Source: three-view drawing plus pictorial views. Frame: mm from the lowest corner of the part. A direction names the side the tool comes from. Coordinates: 2 decimals unless noted, no trailing zeros. Write each loop counter-clockwise with the first axis right and the second up, starting at its lowest first coordinate (ties: lowest second). Pieces come first, ordered by that corner, then holes. Notation, with made-up numbers: (-36.5, 71) - (5.5, 71) arc R11 cw to (5.5, 75) - close; hole circle Ø3 at (17.25, 50). An arc over 180 degrees is marked (long way). One line per item, written item: value.
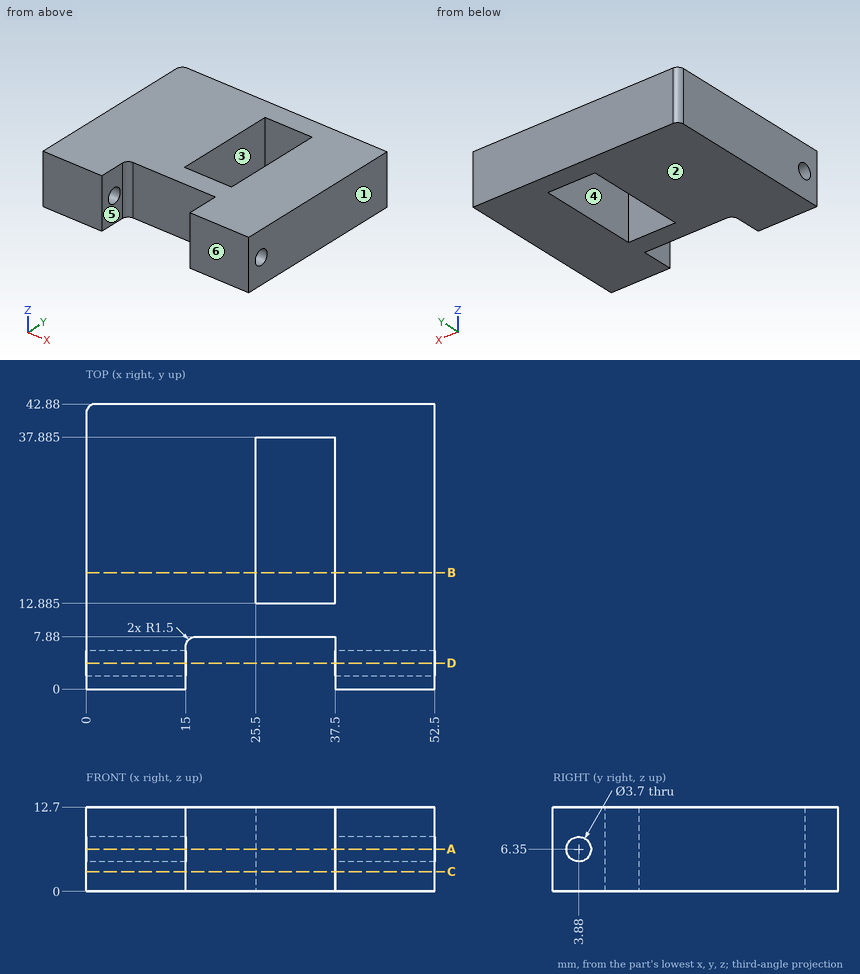
1) Draft query along X for the marked faces 1, 2 and 3. Return one class per face: released by +X, released by -X, zero draft, split by the parting line, or undercut.
Values found:
face 1: released by +X
face 2: zero draft
face 3: undercut
2) Section query B-B on y = 17.5. Output: boundary loops of the cut face in (x, z).
Values found:
outline: (0, 0) - (25.5, 0) - (25.5, 12.7) - (0, 12.7) - close; (37.5, 0) - (52.5, 0) - (52.5, 12.7) - (37.5, 12.7) - close
3) Contact query for flat-ended pins moving along their axis: P1, Ø6, axis at x = 32, z = 3, coming from the -Y side; P2, Ø6, axis at y = 18, z = 10, coming from the -X side. Output: stop coordinate, or through.
Values found:
P1: y = 7.88
P2: x = 0
4) Reachability of the marked faces 4, 5 and 6 from +Z, -Z, +X, -X, +Y, -Y: full face, straight path, thin tool, end or side. Return the list, or none.
Values found:
face 4: +Z, -Z
face 5: +Z, -Z, -Y
face 6: +Z, -Z, +X, -X, -Y
5) Section query D-D on y = 3.88. Output: boundary loops of the cut face in (x, z), then the cut area to 3 significant figures.
Values found:
outline: (0, 0) - (15, 0) - (15, 4.5) - (0, 4.5) - close; (0, 8.2) - (15, 8.2) - (15, 12.7) - (0, 12.7) - close; (37.5, 0) - (52.5, 0) - (52.5, 4.5) - (37.5, 4.5) - close; (37.5, 8.2) - (52.5, 8.2) - (52.5, 12.7) - (37.5, 12.7) - close
area: 270 mm2
6) Section query C-C on z = 3. Output: boundary loops of the cut face in (x, y) (3 decimals).
Values found:
outline: (0, 0) - (15, 0) - (15, 6.38) arc R1.5 cw to (16.5, 7.88) - (37.5, 7.88) - (37.5, 0) - (52.5, 0) - (52.5, 42.88) - (1.5, 42.88) arc R1.5 ccw to (0, 41.38) - close; hole (25.5, 12.885) - (37.5, 12.885) - (37.5, 37.885) - (25.5, 37.885) - close
7) Material intervals for line 1 (X direction, y = 16.5, z = 8.5); line 2 (Z direction, x = 3.5, y = 3.88); line 3 (Y direction, x = 27, z = 10.5) (3 decimals), sorted ascending.
Values found:
line 1: 0 to 25.5, 37.5 to 52.5
line 2: 0 to 4.5, 8.2 to 12.7
line 3: 7.88 to 12.885, 37.885 to 42.88
8) Section query A-A on z = 6.35. Output: boundary loops of the cut face in (x, y) (3 decimals), then the cut area to 3 significant figures.
Values found:
outline: (0, 0) - (15, 0) - (15, 2.03) - (0, 2.03) - close; (0, 5.73) - (15, 5.73) - (15, 6.38) arc R1.5 cw to (16.5, 7.88) - (37.5, 7.88) - (37.5, 5.73) - (52.5, 5.73) - (52.5, 42.88) - (1.5, 42.88) arc R1.5 ccw to (0, 41.38) - close; (37.5, 0) - (52.5, 0) - (52.5, 2.03) - (37.5, 2.03) - close; hole (25.5, 12.885) - (37.5, 12.885) - (37.5, 37.885) - (25.5, 37.885) - close
area: 1,660 mm2
